Could you check a few things on this drawing? It's one solid part, dimensions in mm from its lowest x, y, z. A direction names the side the tool comes from. Coordinates: 2 decimals unless noted, no trailing zeros. Write each loop counter-clockwise with the first axis right and the second up, starting at its lowest first coordinate (ties: lowest second). Pieces come first, ordered by that corner, then holes. Notation, with made-up numbers: M -12,52 L 33,52 A14 ccw 33,71 Z; hole C 28.25,56 d10. An arc over 180 degrees is marked long. Use a Markdown table: item, result.
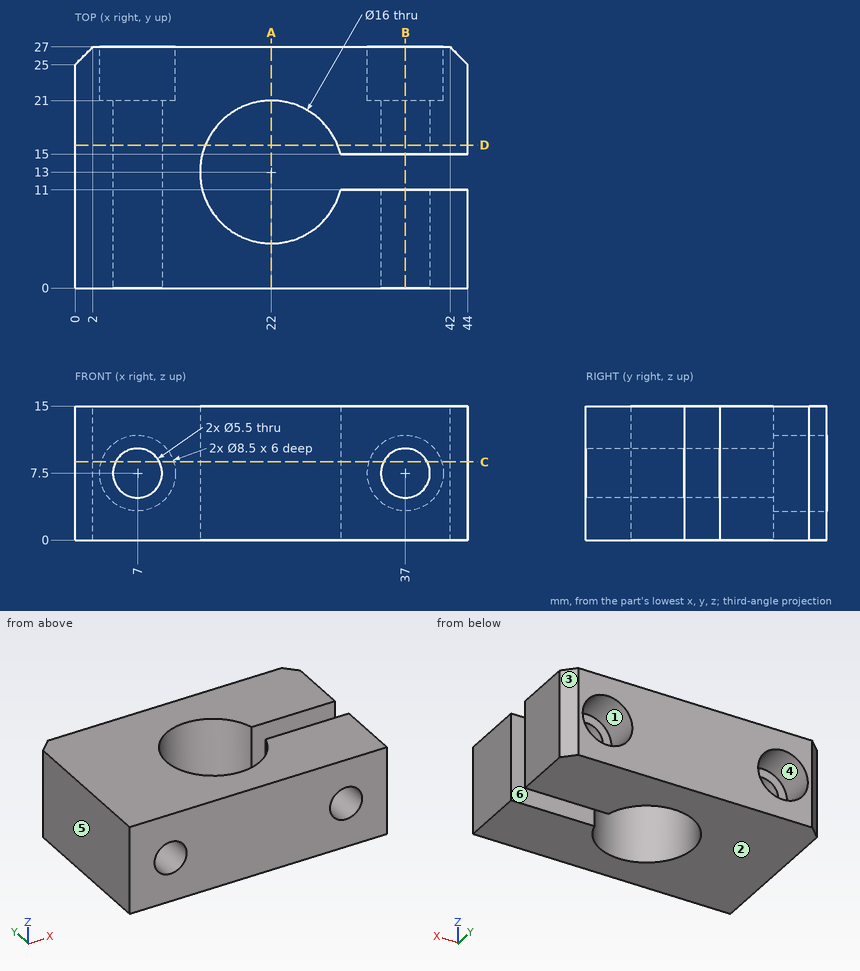
1. Which directions (+Z, -Z, +X, -X, +Y, -Y) give clear straight access to the entire face, cutting with the end or side of a thin tool? Please do the marked faces 4, 5 and 6.
Answers follow:
| item | result |
|---|---|
| face 4 | +Y |
| face 5 | +Z, -Z, -X, +Y, -Y |
| face 6 | +Z, -Z, +X |
2. Suppose I cut it at C-C on z = 8.75. State how many separate pieces and enclosed holes the cut face has, and give its area (3 significant figures).
Answers follow:
| item | result |
|---|---|
| separate pieces | 4 |
| enclosed holes | 0 |
| area | 643 mm2 |
3. We'd pull the mould along Z, two halves only. Please class the marked faces 1, 2 and 3: +Z half, -Z half, draft (parallel to the pull), parting line (faces both ways), or undercut.
Answers follow:
| item | result |
|---|---|
| face 1 | undercut |
| face 2 | -Z half |
| face 3 | draft |
4. Suppose I cut it at D-D on y = 16. Write out the boundary of the cut face in (x, z).
Answers follow:
| item | result |
|---|---|
| outline | M 0,0 L 14.58,0 L 14.58,15 L 0,15 Z; M 29.42,0 L 44,0 L 44,15 L 29.42,15 Z; hole C 7,7.5 d5.5; hole C 37,7.5 d5.5 |
5. Suppose I cut it at A-A on x = 22. Write out the boundary of the cut face in (y, z), and give its area (3 significant figures).
Answers follow:
| item | result |
|---|---|
| outline | M 0,0 L 5,0 L 5,15 L 0,15 Z; M 21,0 L 27,0 L 27,15 L 21,15 Z |
| area | 165 mm2 |
6. Will this pin go through, and if not, where does the flat tip stop? pin 1 Ø4 at (x, z) = (37, 9) entering from +Y.
Answers follow:
| item | result |
|---|---|
| pin 1 | stops at y = 21 |
7. Suppose I cut it at B-B on x = 37. Write out the boundary of the cut face in (y, z), and give its area (4 significant figures).
Answers follow:
| item | result |
|---|---|
| outline | M 0,0 L 11,0 L 11,4.75 L 0,4.75 Z; M 0,10.25 L 11,10.25 L 11,15 L 0,15 Z; M 15,0 L 27,0 L 27,3.25 L 21,3.25 L 21,4.75 L 15,4.75 Z; M 15,10.25 L 21,10.25 L 21,11.75 L 27,11.75 L 27,15 L 15,15 Z |
| area | 200.5 mm2 |
8. I need wall thicknesses on probe 1 along Y at (x, z) = (33.5, 11.5); probe 2 along Z at (x, y) = (37, 24.9); probe 3 along X at (y, z) = (4, 5.75). Which ranges of each line are inside material? Lowest first, please.
Answers follow:
| item | result |
|---|---|
| probe 1 | y = 0 to 11, 15 to 27 |
| probe 2 | z = 0 to 3.25, 11.75 to 15 |
| probe 3 | x = 0 to 4.88, 9.12 to 34.88, 39.12 to 44 |
